Verification items for this drawing (mm, ordinates from the low corner). Round coordinates to 2 decimals unless told otherwise and drop trailing zeros. Order: outer loops, then holes, each group sorted by start corner. A loop starts at its lowest first (then second) coordinate and runs counter-clockwise, first axis right, second up. Notation, with made-up numbers: M 71.25,61.5 L 95.25,61.5 A19 cw 95.25,90.5 Z; hole C 28.25,74.25 d3. An arc over 180 degrees is marked long. Return JSON: item names as keys, results as strings. Group by question number.
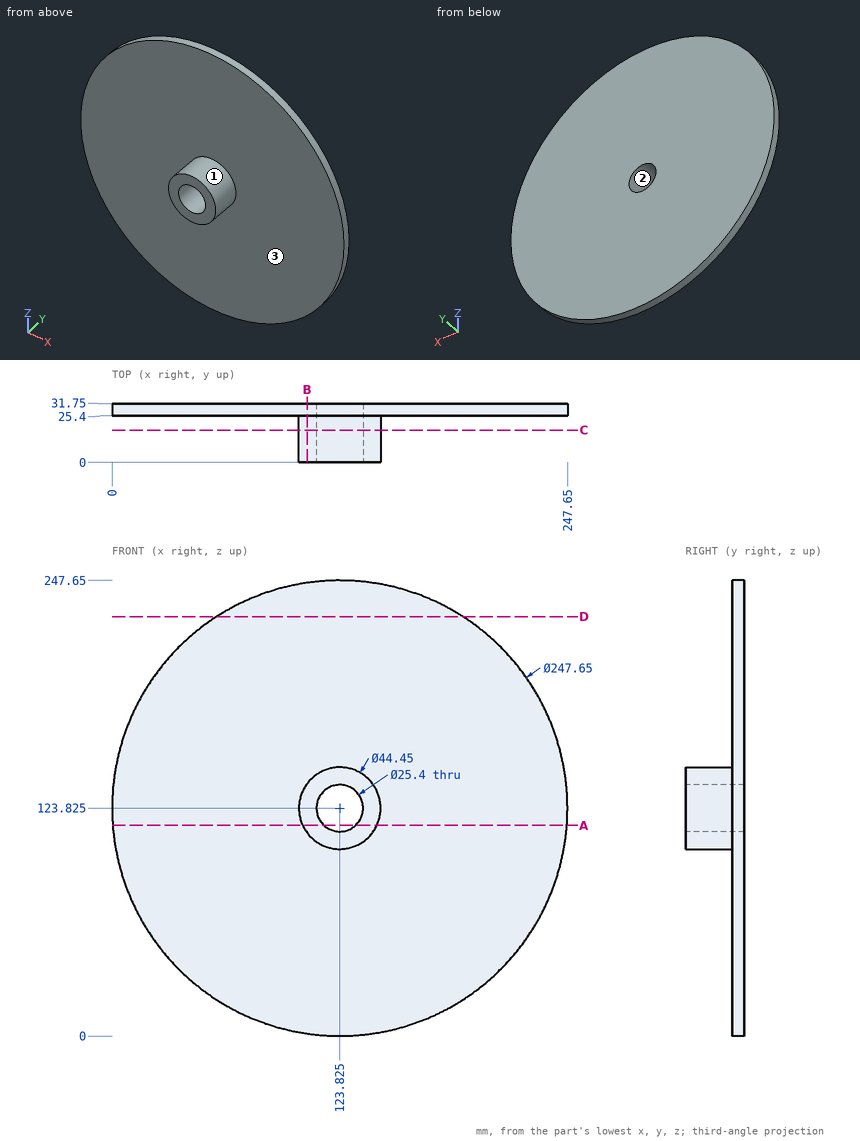
1. Cross-section at C-C (y = 17.5). Enter the section's corners in (x, z) (3 decimals), plus the area to 3 significant figures.
2. Go/stop test with flat-tipped pins: pin 1 (10 mm diameter, centred on x = 94.5, z = 106.5, fed in from -Y); pin 2 (6 mm diameter, centred on x = 44, y = 27.5, fed in from +Z); pin 3 (2 mm diameter, centred on x = 128, y = 21, fed in from -Z). Record where each tip stops, or that it passes through.
3. Cross-section at B-B (x = 106). Enter the section's corners in (y, z), plus the area to 3 significant figures.
4. Draft check along X on the marked faces 1, 2 and 3. Enter one of: +X half, -X half, draft (parallel to the pull), parting line (faces both ways), or undercut.
5. Cross-section at D-D (z = 228). Enter the section's corners in (x, y).
6. Cross-section at A-A (z = 114.5). Enter the section's corners in (x, y), plus the area to 3 significant figures.
7. Thickness scan on line 1 along Y through (x, z) = (122.5, 188.5); line 2 along X through (y, z) = (4, 112.5); line 3 along Z through (x, y) = (121, 15). Record the ranges inside material, lowest first. Write a range as from..to.
Computed:
{
 "1": {"outline": "C 123.825,123.825 d44.45; hole C 123.825,123.825 d25.4", "area": "1,050 mm²"},
 "2": {"pin 1": "stops at y = 25.4", "pin 2": "stops at z = 220.94", "pin 3": "stops at z = 101.83"},
 "3": {"outline": "M 0,110.55 L 25.4,110.55 L 25.4,1.29 L 31.75,1.29 L 31.75,246.36 L 25.4,246.36 L 25.4,137.1 L 0,137.1 Z", "area": "2,230 mm²"},
 "4": {"face 1": "parting line", "face 2": "undercut", "face 3": "draft"},
 "5": {"outline": "M 56.89,25.4 L 190.76,25.4 L 190.76,31.75 L 56.89,31.75 Z"},
 "6": {"outline": "M 0.35,25.4 L 103.65,25.4 L 103.65,0 L 115.2,0 L 115.2,31.75 L 0.35,31.75 Z; M 132.45,0 L 144,0 L 144,25.4 L 247.3,25.4 L 247.3,31.75 L 132.45,31.75 Z", "area": "2,050 mm²"},
 "7": {"line 1": "y = 25.4..31.75", "line 2": "x = 104.7..118.08, 129.57..142.95", "line 3": "z = 101.78..111.44, 136.21..145.87"}
}
